from build123d import *

# Parameters (mm, degrees)
BOSS_EXTRUDE1_DEPTH  = 5
SKETCH2_W            = 160
SKETCH2_H            = 200
BOSS_EXTRUDE2_DEPTH  = 5
SKETCH4_W            = 160
SKETCH4_H            = 190
BOSS_EXTRUDE4_DEPTH  = 5
SKETCH5_W            = 160
SKETCH5_H            = 90
BOSS_EXTRUDE5_DEPTH  = 5
SKETCH6_W            = 96
SKETCH6_H            = 39
SKETCH6_W_2          = 11
SKETCH6_H_2          = 11
CUT_EXTRUDE2_DEPTH   = 5
FILLET1_R            = 40
SKETCH7_W            = 70
SKETCH7_H            = 77
CUT_EXTRUDE3_DEPTH   = 1
SKETCH8_W            = 22
SKETCH8_H            = 4
CUT_EXTRUDE4_DEPTH   = 4
SKETCH9_W            = 40
SKETCH9_H            = 60
CUT_EXTRUDE5_DEPTH   = 5
SKETCH12_W           = 40
SKETCH12_H           = 60
BOSS_EXTRUDE6_DEPTH  = 2
SKETCH14_W           = 77
SKETCH14_H           = 53
CUT_EXTRUDE6_DEPTH   = 5
SKETCH15_W           = 3
SKETCH15_H           = 29
CUT_EXTRUDE7_DEPTH   = 5
SKETCH17_R           = 1.75
CUT_EXTRUDE9_DEPTH   = 4
SKETCH21_R           = 1.5
BOSS_EXTRUDE8_DEPTH  = 4
SKETCH23_R           = 1.5
BOSS_EXTRUDE9_DEPTH  = 10
SKETCH25_R           = 1.5
BOSS_EXTRUDE10_DEPTH = 10


with BuildPart() as part:
    # Sketch1 → Boss-Extrude1 (new body)
    with BuildSketch(Plane(origin=(0, 0, 0), x_dir=(0, 0, -1), z_dir=(1, 0, 0))):
        Polygon((0, 0), (173.205080757, -100), (173.205080757, -190), (0, -190), align=None)
    boss_extrude1 = extrude(amount=BOSS_EXTRUDE1_DEPTH)

    # Sketch2 → Boss-Extrude2 (add)
    with BuildSketch(Plane(origin=(0, 0, 0), x_dir=(1, 0, 0), z_dir=(0, 0.8660254037844382, -0.5000000000000011))):
        with Locations((80, 100)):
            Rectangle(SKETCH2_W, SKETCH2_H)
    extrude(amount=-BOSS_EXTRUDE2_DEPTH)

    # Sketch4 → Boss-Extrude4 (add)
    with BuildSketch(Plane.XY):
        with Locations((80, -95)):
            Rectangle(SKETCH4_W, SKETCH4_H)
    extrude(amount=BOSS_EXTRUDE4_DEPTH)

    # Sketch5 → Boss-Extrude5 (add)
    with BuildSketch(Plane(origin=(0, 0, -173.205080757), x_dir=(-1, 0, 0), z_dir=(0, 0, -1))):
        with Locations((-80, -145)):
            Rectangle(SKETCH5_W, SKETCH5_H)
    extrude(amount=-BOSS_EXTRUDE5_DEPTH)

    # Mirror1: Boss-Extrude1 across plane
    add(boss_extrude1.mirror(Plane.ZY.offset(-80)))

    # Sketch6 → Cut-Extrude2 (cut)
    with BuildSketch(Plane(origin=(0, 0, 0), x_dir=(1, 0, 0), z_dir=(0, 0.8660254037844382, -0.5000000000000011))):
        with Locations((102, 36.815172727)):
            Rectangle(SKETCH6_W, SKETCH6_H)
        with Locations((34, 15.815172727)):
            Rectangle(SKETCH6_W_2, SKETCH6_H_2)
        with Locations((34, 36.815172727)):
            Rectangle(SKETCH6_W_2, SKETCH6_H_2)
        with Locations((34, 57.815172727)):
            Rectangle(SKETCH6_W_2, SKETCH6_H_2)
    extrude(amount=-CUT_EXTRUDE2_DEPTH, mode=Mode.SUBTRACT)

    # Fillet1
    fillet1_edges = [part.edges().sort_by_distance(p)[0] for p in [
        (80, -100, -173.205080757),
    ]]
    fillet(fillet1_edges, radius=FILLET1_R)

    # Sketch7 → Cut-Extrude3 (cut)
    with BuildSketch(Plane(origin=(0, 0, 0), x_dir=(1, 0, 0), z_dir=(0, 0.8660254037844382, -0.5000000000000011))):
        with Locations((105, 121.815172727)):
            Rectangle(SKETCH7_W, SKETCH7_H)
    extrude(amount=-CUT_EXTRUDE3_DEPTH, mode=Mode.SUBTRACT)

    # Sketch8 → Cut-Extrude4 (cut)
    with BuildSketch(Plane(origin=(0, -0.866025403784426, 0.4999999999999943), x_dir=(1, 0, 0), z_dir=(0, 0.8660254037844382, -0.5000000000000011))):
        with Locations((105, 158.315172727)):
            Rectangle(SKETCH8_W, SKETCH8_H)
    extrude(amount=-CUT_EXTRUDE4_DEPTH, mode=Mode.SUBTRACT)

    # Sketch9 → Cut-Extrude5 (cut)
    with BuildSketch(Plane(origin=(0, 0, 0), x_dir=(1, 0, 0), z_dir=(0, 0.8660254037844382, -0.5000000000000011))):
        with Locations((35, 121.815172727)):
            Rectangle(SKETCH9_W, SKETCH9_H)
    extrude(amount=-CUT_EXTRUDE5_DEPTH, mode=Mode.SUBTRACT)

    # Sketch12 → Boss-Extrude6 (add)
    with BuildSketch(Plane(origin=(0, 0, 0), x_dir=(1, 0, 0), z_dir=(0, 0.8660254037844382, -0.5000000000000011))):
        with Locations((35, 121.815172727)):
            Rectangle(SKETCH12_W, SKETCH12_H)
    extrude(amount=-BOSS_EXTRUDE6_DEPTH)

    # Sketch14 → Cut-Extrude6 (cut)
    with BuildSketch(Plane(origin=(0, 0, -173.205080757), x_dir=(-1, 0, 0), z_dir=(0, 0, -1))):
        with Locations((-101.5, -156.594010768)):
            Rectangle(SKETCH14_W, SKETCH14_H)
    extrude(amount=-CUT_EXTRUDE6_DEPTH, mode=Mode.SUBTRACT)

    # Sketch15 → Cut-Extrude7 (cut)
    with BuildSketch(Plane(origin=(0, 0, -173.205080757), x_dir=(-1, 0, 0), z_dir=(0, 0, -1))):
        with Locations((-61.5, -156.594010768)):
            Rectangle(SKETCH15_W, SKETCH15_H)
        with Locations((-141.5, -156.594010768)):
            Rectangle(SKETCH15_W, SKETCH15_H)
    extrude(amount=-CUT_EXTRUDE7_DEPTH, mode=Mode.SUBTRACT)

    # Sketch17 → Cut-Extrude9 (cut)
    with BuildSketch(Plane(origin=(0, -4.330127019, 2.5), x_dir=(-1, 0, 0), z_dir=(0, -0.8660254037844382, 0.500000000000001))):
        with Locations(Location((-54.75, 64.989476433, 0), (0, 0, 90))):
            Circle(SKETCH17_R)
        with Locations(Location((-149.25, 64.989476433, 0), (0, 0, 270))):
            Circle(SKETCH17_R)
        with Locations(Location((-54.75, 8.489476433, 0), (0, 0, 270))):
            Circle(SKETCH17_R)
        with Locations(Location((-149.25, 8.489476433, 0), (0, 0, 90))):
            Circle(SKETCH17_R)
    extrude(amount=-CUT_EXTRUDE9_DEPTH, mode=Mode.SUBTRACT)

    # Sketch21 → Boss-Extrude8 (add)
    with BuildSketch(Plane(origin=(0, -1.732050808, 1), x_dir=(-1, 0, 0), z_dir=(0, -0.8660254037844382, 0.500000000000001))):
        with Locations(Location((-48.5, 98.315172727, 0), (0, 0, 270))):
            Circle(SKETCH21_R)
        with Locations(Location((-21.5, 97.315172727, 0), (0, 0, 270))):
            Circle(SKETCH21_R)
        with Locations(Location((-17.5, 136.315172727, 0), (0, 0, 270))):
            Circle(SKETCH21_R)
        with Locations(Location((-52.5, 136.315172727, 0), (0, 0, 270))):
            Circle(SKETCH21_R)
    extrude(amount=BOSS_EXTRUDE8_DEPTH)

    # Sketch23 → Boss-Extrude9 (add)
    with BuildSketch(Plane(origin=(0, -190, 0), x_dir=(-1, 0, 0), z_dir=(0, -1, 0))):
        with BuildLine():
            Line((-155, 0), (-145, 0))
            ThreePointArc((-145, 0), (-147.928932188, 7.071067812), (-155, 10))
            Line((-155, 10), (-155, 0))
        make_face()
        with Locations(Location((-151.751738587, 3.801157428, 0), (0, 0, 90))):
            Circle(SKETCH23_R, mode=Mode.SUBTRACT)
    boss_extrude9 = extrude(amount=-BOSS_EXTRUDE9_DEPTH)

    # Mirror2: Boss-Extrude9 across plane
    add(boss_extrude9.mirror(Plane.ZY.offset(-80)))

    # Sketch25 → Boss-Extrude10 (add)
    with BuildSketch(Plane(origin=(0, -190, 0), x_dir=(-1, 0, 0), z_dir=(0, -1, 0))):
        with BuildLine():
            Line((-155, 168.205080757), (-145, 168.205080757))
            ThreePointArc((-145, 168.205080757), (-147.928932188, 161.134012945), (-155, 158.205080757))
            Line((-155, 158.205080757), (-155, 168.205080757))
        make_face()
        with Locations(Location((-151.620258089, 164.520335906, 0), (0, 0, 90))):
            Circle(SKETCH25_R, mode=Mode.SUBTRACT)
    boss_extrude10 = extrude(amount=-BOSS_EXTRUDE10_DEPTH)

    # Mirror4: Boss-Extrude10 across plane
    add(boss_extrude10.mirror(Plane.ZY.offset(-80)))


solid = part.part
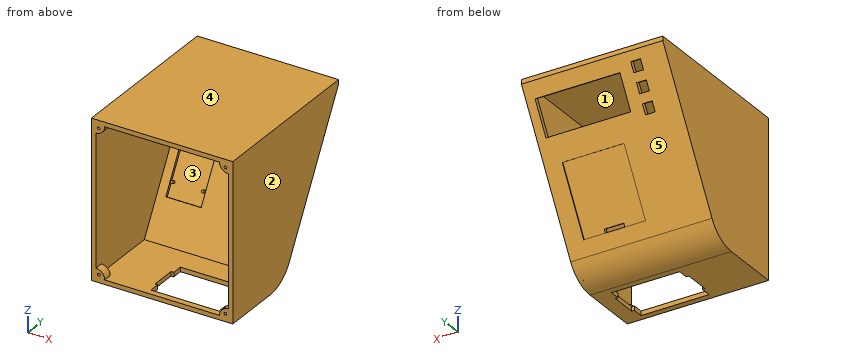
Geometry check sheet. Reference: the model listing, model coordinates, mm. Face numbers are marked on the shaded views. A direction names the side the tool comes from. Coordinates: 2 decimals unless noted, no trailing zeros. Loops run counter-clockwise (first coordinate to the right, second up) from the corner with the lowest first, then second, coordinate; pieces in that order, holes last. Notation, with made-up numbers: (64, 6) - (109, 6) arc R31 ccw to (109, 44) - close; hole circle Ø1 at (87, 88). An arc over 180 degrees is marked (long way). Use one line per item in the form item = value. Start each with the question number.
Item 1: Gauge pin test, flat ends, axial feed: pin 1 (1 mm diameter, centred on x = 137.5, z = -59, fed in from -Y); pin 2 (5 mm diameter, centred on x = 122, z = -134, fed in from -Y); pin 3 (4 mm diameter, centred on x = 47, z = -112.5, fed in from +Y). Record the tip position at first contact, or that the pin passes through.
Item 2: Section check A-A, the plane z = -40. Enter the section's corners in (x, y).
Item 3: Section check C-C, the plane y = -161. Enter the section's corners in (x, z), and give its area (3 significant figures).
Item 4: Mould release check, pull along Z, two halves, no side actions. Record for the marked faces 3, 4 and 5: +Z half, -Z half, draft (parallel to the pull), parting line (faces both ways), or undercut.
Item 5: Thickness scan on probe 1 along X at (y, z) = (-47, -41); probe 2 along Z at (x, y) = (145.5, -65); probe 3 along Z at (x, y) = (144, -11). Record the ranges inside material, lowest first.
Item 6: Tool access check on the marked faces 1 and 2. Record the directions out of +Z, -Z, +X, -X, +Y, -Y that give a thin tool (end or side, any length) a straight path to the whole face; none if there is none.
Computed:
q1.pin_1 = -40.13
q1.pin_2 = -84.58
q1.pin_3 = -63.8
q2.outline = (0, -190) - (5, -190) - (5, -28.87) - (54, -28.87) - (54, -23.09) - (0, -23.09) - close; (150, -28.87) - (155, -28.87) - (155, -190) - (160, -190) - (160, -23.09) - (150, -23.09) - close
q3.outline = (0, -173.21) - (60, -173.21) - (60, -168.21) - (5, -168.21) - (5, 0) - (155, 0) - (155, -168.21) - (143, -168.21) - (143, -173.21) - (160, -173.21) - (160, 5) - (0, 5) - close
q3.area = 2,870 mm2
q4.face_3 = undercut
q4.face_4 = +Z half
q4.face_5 = -Z half
q5.probe_1 = 0 to 5, 155 to 160
q5.probe_2 = -112.58 to -102.58, 0 to 5
q5.probe_3 = -13.64 to -9.05, 0 to 5
q6.face_1 = none
q6.face_2 = +Z, -Z, +X, +Y, -Y
